Could you check a few things on this model? Use its own coordinates, in mm. Face numbers are marked on the shaded views. A direction names the side the tool comes from. Give positions to 0.01 mm unless a question says otherwise; leave off trailing zeros. Loops run counter-clockwise (first coordinate to the right, second up) from the corner with the lowest first, then second, coordinate; pieces in that order, holes last. Notation, with made-up numbers: (-21, 0.25) - (10, 0.25) arc R27 cw to (10, 30.25) - close; hole circle Ø3 at (51.5, 47). An arc over 180 degrees is marked (long way). Answer in a Markdown table with one row per item. Add a question column.
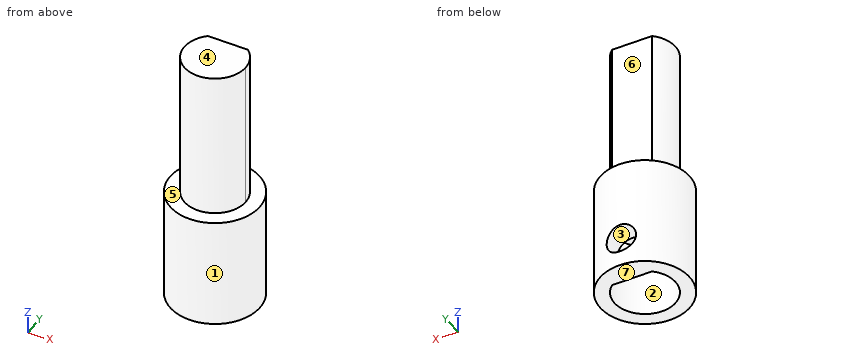
```python
from build123d import *

# Parameters (mm, degrees)
SKETCH1_R                = 6
BOSS_EXTRUDE1_DEPTH      = 15
BOSS_EXTRUDE2_DEPTH      = 20
BOSS_EXTRUDE2_DEPTH_BACK = 5
BOSS_EXTRUDE2_START      = 15
CUT_EXTRUDE1_REACH       = 38.014
CUT_EXTRUDE1_END_RADIUS  = 6
SKETCH3_R                = 1.975


with BuildPart() as part:
    # Sketch1 → Boss-Extrude1 (new body)
    with BuildSketch(Plane.XY):
        Circle(SKETCH1_R)
        with BuildLine():
            Line((-2.683281573, 3.1), (2.683281573, 3.1))
            ThreePointArc((2.683281573, 3.1), (0, -4.1), (-2.683281573, 3.1))
        make_face(mode=Mode.SUBTRACT)
    extrude(amount=BOSS_EXTRUDE1_DEPTH)

    # Sketch1<3> → Boss-Extrude2 (add, two sides: drawn at the far end of the back side and taken through both)
    with BuildSketch(Plane.XY.offset(BOSS_EXTRUDE2_START - BOSS_EXTRUDE2_DEPTH_BACK)):
        with BuildLine():
            Line((2.683281573, 3.1), (-2.683281573, 3.1))
            ThreePointArc((-2.683281573, 3.1), (-1.704192705, -3.729038378), (4.1, 0))
            ThreePointArc((4.1, 0), (3.729038378, 1.704192705), (2.683281573, 3.1))
        make_face()
    extrude(amount=BOSS_EXTRUDE2_DEPTH + BOSS_EXTRUDE2_DEPTH_BACK)

    # Cut-Extrude1: up to this cylinder (the profile starts inside it)
    cut_extrude1_end = Plane(origin=(0, 0, 4), z_dir=(0, 0, -1)) * Cylinder(CUT_EXTRUDE1_END_RADIUS, 89.028, mode=Mode.PRIVATE)
    # Sketch3 → Cut-Extrude1 (cut, up to the surface)
    with BuildSketch(Plane(origin=(0, 0, 0), x_dir=(1, 0, 0), z_dir=(0, 1, 0)), mode=Mode.PRIVATE) as cut_extrude1_sk1:
        with Locations(Location((0, -4, 0), (0, 0, 90))):
            Circle(SKETCH3_R)
    cut_extrude1_tool1 = extrude(cut_extrude1_sk1.sketch, amount=CUT_EXTRUDE1_REACH, mode=Mode.PRIVATE) & cut_extrude1_end
    add(cut_extrude1_tool1.solids().sort_by_distance((0, 0, 4))[0], mode=Mode.SUBTRACT)


solid = part.part
```
(1) We'd pull the mould along X, two halves only. Please class the marked faces 1, 2, 3 and 4: pulls with the +X half, pulls with the -X half, needs draft (parallel to the pull), parting line crosses it, or undercut.
(2) For pin 1 Ø2.5 at (x, z) = (-1, 24) entering from +Y; pin 2 Ø6 at (x, z) = (-3.5, 7) entering from +Y; pin 3 Ø1 at (y, z) = (1, 6.5) entering from -X, each with a flat end and sliding along its axis, tell me the tip position at first contact or that it passes through.
(3) On a 3-axis mill with a long thin cutter (end or side, diameter ignored), from which of +Z, -Z, +X, -X, +Y, -Y can I reach the whole of each face in a straight line? I mean the marked faces 5, 6 and 7. Say none if no direction works.
(4) I want a section at A-A on x = 0. Please give me the cut outline in (y, z) (3 decimals), then the cut area to 3 significant figures.
(5) Please list where these lines run through material, in increasing order: line 1 (Z direction, x = -2.5, y = -4.75); line 2 (Y direction, x = 0, z = 5.5); line 3 (Z direction, x = -1, y = 1).
(6) I want a section at B-B on y = 2. Please give me the cut outline in (x, z), then the cut area to 3 significant figures.
(7) I want a section at D-D on x = -3. Please give me the cut outline in (y, z).
(8) I want a section at C-C on z = 6.5. Please give me the cut outline in (x, y).
Reported:
| question | item | result |
|---|---|---|
| 1 | face 1 | parting line crosses it |
| 1 | face 2 | undercut |
| 1 | face 3 | undercut |
| 1 | face 4 | needs draft |
| 2 | pin 1 | y = 3.1 |
| 2 | pin 2 | y = 5.98 |
| 2 | pin 3 | x = -5.98 |
| 3 | face 5 | +Z |
| 3 | face 6 | +Z, +X, -X, +Y |
| 3 | face 7 | -Z, +X, -X, +Y, -Y |
| 4 | outline | (-6, 0) - (-4.1, 0) - (-4.1, 10) - (3.1, 10) - (3.1, 5.975) - (6, 5.975) - (6, 15) - (3.1, 15) - (3.1, 35) - (-4.1, 35) - (-4.1, 15) - (-6, 15) - close; (3.1, 0) - (6, 0) - (6, 2.025) - (3.1, 2.025) - close |
| 4 | area | 241 mm² |
| 5 | line 1 | 0 to 15 |
| 5 | line 2 | -6 to -4.1 |
| 5 | line 3 | 10 to 35 |
| 6 | outline | (-5.66, 0) - (-3.58, 0) - (-3.58, 10) - (3.58, 10) - (3.58, 0) - (5.66, 0) - (5.66, 15) - (3.58, 15) - (3.58, 35) - (-3.58, 35) - (-3.58, 15) - (-5.66, 15) - close |
| 6 | area | 241 mm² |
| 7 | outline | (-5.2, 0) - (-2.79, 0) - (-2.79, 10) - (2.79, 10) - (2.79, 0) - (5.2, 0) - (5.2, 15) - (2.79, 15) - (2.79, 35) - (-2.79, 35) - (-2.79, 15) - (-5.2, 15) - close |
| 8 | outline | circle Ø12 at (0, 0); hole (-2.68, 3.1) arc R4.1 ccw (long way) to (2.68, 3.1) - close |
